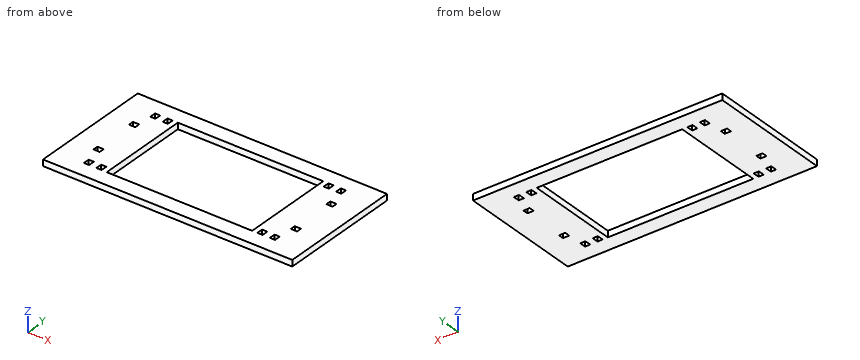
Autodesk Fusion 360 part; units mm, degrees
sketch "Sketch1" plane through (0, 0, 0) normal (0, 0, 1) x (1, 0, 0) in component "Base"
  line L0 (120, 60) -> (-120, 60)
  line L1 (-120, 60) -> (-120, -60)
  line L2 (-120, -60) -> (120, -60)
  line L3 (120, -60) -> (120, 60)
  line L4 (120, 60) -> (-120, -60) construction
  line L5 (-120, 60) -> (120, -60) construction
  line L6 (-70, 45) -> (70, 45)
  line L7 (70, 45) -> (70, -45)
  line L8 (70, -45) -> (-70, -45)
  line L9 (-70, -45) -> (-70, 45)
  line L10 (-70, 45) -> (70, -45) construction
  line L11 (70, 45) -> (-70, -45) construction
  dimension "d1" = 240
  dimension "d2" = 120
  dimension "d3" = 90
  dimension "d6" = 140
extrude "Extrude1" add sketch "Sketch1" along normal blind 6 in component "Base"
sketch "Sketch2" plane through (0, 0, 6) normal (0, 0, 1) x (-1, 0, 0) in component "Base"
  line L0 (-70, 45) -> (70, 45)
  line L1 (70, 45) -> (70, -45)
  line L2 (70, -45) -> (-70, -45)
  line L3 (-70, -45) -> (-70, 45)
  line L4 (-120, 60) -> (-120, -60)
  line L5 (-120, -60) -> (120, -60)
  line L6 (120, -60) -> (120, 60)
  line L7 (120, 60) -> (-120, 60)
  line L8 (70, 45) -> (92, 45) construction
  line L9 (92, 45) -> (92, 39) construction
  line L10 (92, 39) -> (70, 39) construction
  line L11 (70, 39) -> (70, 45) construction
  line L12 (92, 39) -> (87, 39)
  line L13 (87, 39) -> (87, 45)
  line L14 (87, 45) -> (92, 45)
  line L15 (92, 45) -> (92, 39)
  line L16 (70, 39) -> (75, 39) construction
  line L17 (75, 45) -> (75, 39) construction
  line L18 (75, 39) -> (80, 39)
  line L19 (80, 39) -> (80, 45)
  line L20 (80, 45) -> (75, 45)
  line L21 (75, 45) -> (75, 39)
  dimension "d15" = 6
extrude "Extrude2" cut sketch "Sketch2" against normal blind 6 contours L12 L13 L14 L15 | L18 L19 L20 L21 in component "Base"
ref_plane "WorkPlane1" through (0, 0, 0) normal (1, 0, 0) x (0, 1, 0) in component "Base"
mirror "Mirror1" about plane through (0, 0, 0) normal (1, 0, 0) of "Extrude2" in component "Base"
ref_plane "WorkPlane2" through (0, 0, 0) normal (0, 1, 0) x (0, 0, 1) in component "Base"
mirror "Mirror2" about plane through (0, 0, 0) normal (0, 1, 0) of "Extrude2", "Mirror1" in component "Base"
sketch "Sketch3" plane through (0, 0, 0) normal (0, 0, -1) x (1, 0, 0) in component "Base"
  line L0 (87, -45) -> (87, -39)
  line L1 (87, -39) -> (92, -39)
  line L2 (92, -39) -> (92, -45)
  line L3 (92, -45) -> (87, -45)
  line L4 (75, -39) -> (80, -39)
  line L5 (80, -39) -> (80, -45)
  line L6 (80, -45) -> (75, -45)
  line L7 (75, -45) -> (75, -39)
  line L8 (-87, -39) -> (-87, -45)
  line L9 (-87, -45) -> (-92, -45)
  line L10 (-92, -45) -> (-92, -39)
  line L11 (-92, -39) -> (-87, -39)
  line L12 (-80, -39) -> (-75, -39)
  line L13 (-75, -39) -> (-75, -45)
  line L14 (-75, -45) -> (-80, -45)
  line L15 (-80, -45) -> (-80, -39)
  line L16 (87, 39) -> (87, 45)
  line L17 (87, 45) -> (92, 45)
  line L18 (92, 45) -> (92, 39)
  line L19 (92, 39) -> (87, 39)
  line L20 (80, 39) -> (75, 39)
  line L21 (75, 39) -> (75, 45)
  line L22 (75, 45) -> (80, 45)
  line L23 (80, 45) -> (80, 39)
  line L24 (-87, 45) -> (-87, 39)
  line L25 (-87, 39) -> (-92, 39)
  line L26 (-92, 39) -> (-92, 45)
  line L27 (-92, 45) -> (-87, 45)
  line L28 (-75, 39) -> (-80, 39)
  line L29 (-80, 39) -> (-80, 45)
  line L30 (-80, 45) -> (-75, 45)
  line L31 (-75, 45) -> (-75, 39)
  line L32 (-70, 45) -> (70, 45)
  line L33 (70, 45) -> (70, -45)
  line L34 (70, -45) -> (-70, -45)
  line L35 (-70, -45) -> (-70, 45)
  line L36 (120, -60) -> (120, 60)
  line L37 (120, 60) -> (-120, 60)
  line L38 (-120, 60) -> (-120, -60)
  line L39 (-120, -60) -> (120, -60)
  line L40 (-120, 0) -> (-70, 0) construction
  line L41 (-87, -39) -> (-87, 39) construction
  line L42 (-87, 0) -> (-87, -20) construction
  line L43 (-87, 0) -> (-87, -20) construction
  line L44 (-87, 0) -> (-93, 0) construction
  line L45 (-87, 0) -> (-92, 0) construction
  line L46 (-92, 0) -> (-92, -20) construction
  line L47 (-92, -20) -> (-87, -20) construction
  line L48 (-87, -20) -> (-87, 0) construction
  line L49 (-87, 0) -> (-91.9449, 0) construction
  line L50 (-91.9449, 20) -> (-87, 20) construction
  line L51 (-87, 20) -> (-87, 0) construction
  line L52 (-87, 0) -> (-92, 0) construction
  line L53 (-92, 0) -> (-92, 20) construction
  line L54 (-92, 20) -> (-87, 20) construction
  line L55 (-87, 20) -> (-87, 0) construction
  line L56 (-92, -20) -> (-98, -20)
  line L57 (-98, -20) -> (-98, -25)
  line L58 (-98, -25) -> (-92, -25)
  line L59 (-92, -25) -> (-92, -20)
  line L60 (-92, 20) -> (-98, 20)
  line L61 (-98, 20) -> (-98, 25)
  line L62 (-98, 25) -> (-92, 25)
  line L63 (-92, 25) -> (-92, 20)
  dimension "d16" = 5
  dimension "d17" = 20
  dimension "d18" = 20
extrude "Extrude3" cut sketch "Sketch3" against normal blind 11 contours L56 L57 L58 L59 | L60 L61 L62 L63 in component "Base"
mirror "Mirror3" about plane through (0, 0, 0) normal (1, 0, 0) of "Extrude3" in component "Base"
component "Base" placed x (1, 0, 0) y (0, 1, 0) z (0, 0, 1) at (0, 0, 0)
Build history of the part. All positions in model axes, mm. Round coordinates to 2 decimals unless told otherwise and drop trailing zeros. Loops run counter-clockwise (first coordinate to the right, second up) from the corner with the lowest first, then second, coordinate; pieces in that order, holes last. Notation, with made-up numbers: (-17, 8) -> (18, 8) arc R17 ccw to (18, 18) -> close; hole circle Ø6 at (-1.75, -13). An arc over 180 degrees is marked (long way). Use CSV: the item, a comma, the result in double quotes. Start each with the question number.
Q1. Saw through at A-A on x = -1. Give the cut face in (y, z).
Q2. Saw through at B-B on y = -28. Give the cut face in (x, z).
Q3. Drill centre lines: L1, parallel to X at y = -20.5, z = 0.75; L2, parallel to X at y = -32, z = 1.8; L3, parallel to Y at x = -47, z = 5.4. Where is each one in solid material? Low to high.
Q4. Saw through at C-C on z = 2.3. Count the separate pieces of the cut face and the enclosed holes in it, and give its area (3 significant figures).
Solutions:
1,outline,"(-60, 0) -> (-45, 0) -> (-45, 6) -> (-60, 6) -> close; (45, 0) -> (60, 0) -> (60, 6) -> (45, 6) -> close"
2,outline,"(-120, 0) -> (-70, 0) -> (-70, 6) -> (-120, 6) -> close; (70, 0) -> (120, 0) -> (120, 6) -> (70, 6) -> close"
3,L1,"x = -120 to -98, -92 to -70, 70 to 92, 98 to 120"
3,L2,"x = -120 to -70, 70 to 120"
3,L3,"y = -60 to -45, 45 to 60"
4,separate pieces,"1"
4,enclosed holes,"13"
4,area,"15,800 mm^2"
